Design review of the part shown in the three views and the two pictorial views. Dimensions are in mm from the part's minimum x, y and z. A direction names the side the tool comes from. Give positions to 0.01 mm unless a question says otherwise; leave off trailing zeros. Order: outer loops, then holes, each group sorted by start corner. A loop starts at its lowest first (then second) coordinate and runs counter-clockwise, first axis right, second up.
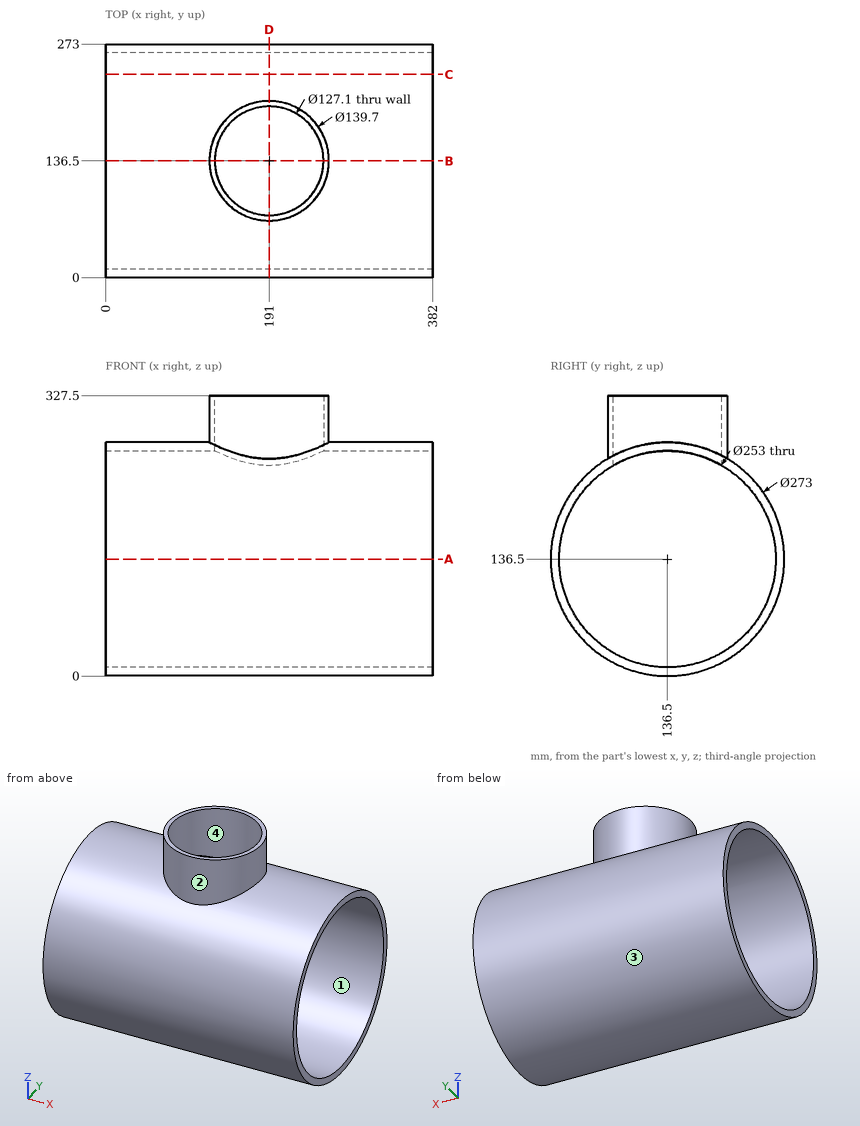
Item 1: Take a section at A-A (z = 136.5). Give the boundary of the cut face in (x, y).
Values found:
outline: (0, 0) - (382, 0) - (382, 10) - (0, 10) - close; (0, 263) - (382, 263) - (382, 273) - (0, 273) - close
Item 2: Draft analysis for pull direction Y (two halves, no side actions). For the marked faces 3 and 4, state which applies: released by +Y, released by -Y, zero draft, split by the parting line, or undercut.
Values found:
face 3: split by the parting line
face 4: undercut
Item 3: For the marked faces 1 and 2, list the 3-axis set-ups (+Z, -Z, +X, -X, +Y, -Y) from which the entire face can be reached by the end or side of a thin tool; tool diameter is ignored.
Values found:
face 1: +X, -X
face 2: +Z
Item 4: Clearance check with flat-ended pins moving along their axes: pin 1 Ø6 at (x, y) = (57.5, 28) entering from +Z; pin 2 Ø6 at (y, z) = (153.5, 280) entering from +X; pin 3 Ø6 at (x, z) = (197, 94) entering from -Y. State where each tip first meets the part, or that it passes through.
Values found:
pin 1: stops at z = 223.11
pin 2: stops at x = 259.43
pin 3: stops at y = 5.84
Item 5: Take a section at D-D (x = 191). Give the boundary of the cut face in (y, z).
Values found:
outline: (66.65, 253.77) arc R136.5 ccw (long way) to (206.35, 253.77) - (206.35, 327.5) - (200.05, 327.5) - (200.05, 245.88) arc R126.5 cw (long way) to (72.95, 245.88) - (72.95, 327.5) - (66.65, 327.5) - close
Item 6: Take a section at C-C (y = 237.5). Give the boundary of the cut face in (x, z).
Values found:
outline: (0, 44.68) - (382, 44.68) - (382, 60.33) - (0, 60.33) - close; (0, 212.67) - (382, 212.67) - (382, 228.32) - (0, 228.32) - close
Item 7: Take a section at B-B (y = 136.5). Give the boundary of the cut face in (x, z).
Values found:
outline: (0, 0) - (382, 0) - (382, 10) - (0, 10) - close; (0, 263) - (127.45, 263) - (127.45, 327.5) - (121.15, 327.5) - (121.15, 273) - (0, 273) - close; (254.55, 263) - (382, 263) - (382, 273) - (260.85, 273) - (260.85, 327.5) - (254.55, 327.5) - close
Item 8: For line 1 (Y direction, x = 248, z = 136); line 2 (Y direction, x = 191, z = 299); line 3 (X direction, y = 136, z = 271), list the stretches that pass through material, from the lowest coordinate up.
Values found:
line 1: y = 0 to 10, 263 to 273
line 2: y = 66.65 to 72.95, 200.05 to 206.35
line 3: x = 0 to 127.45, 254.55 to 382
